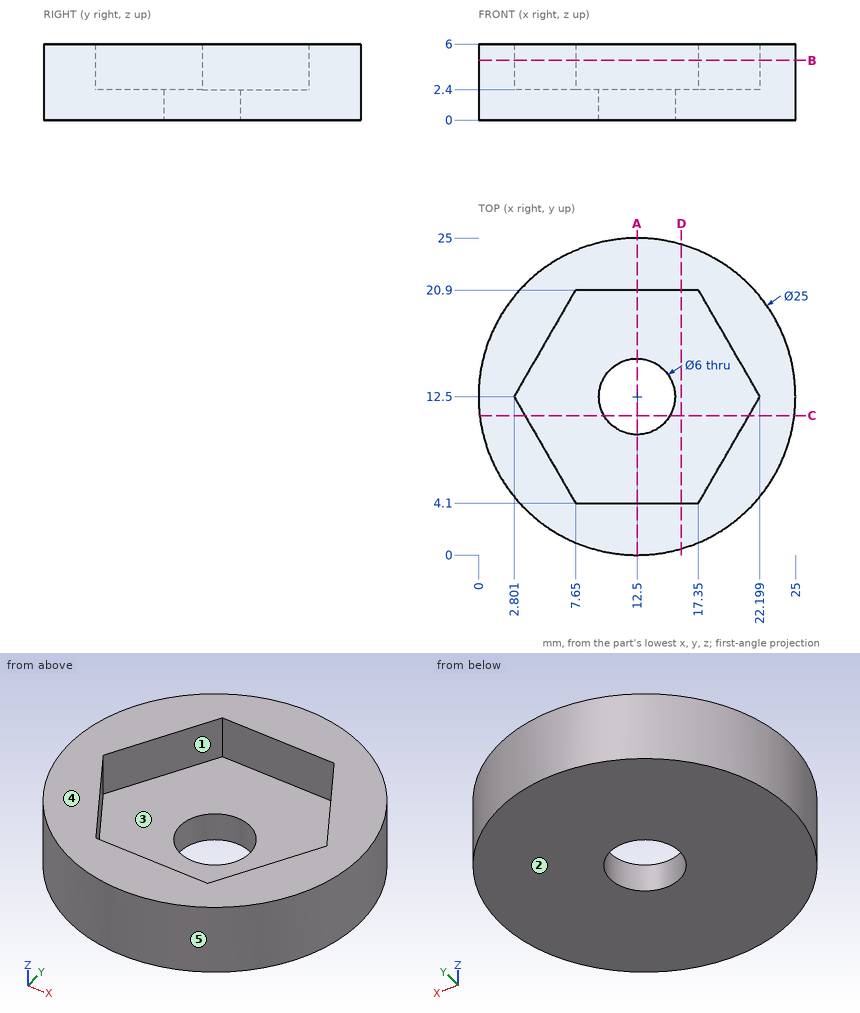
For this review, use the dimensioned drawing (mm, ordinates from the lowest corner) and the shaded views. A direction names the side the tool comes from. Give positions to 0.01 mm unless a question says otherwise; leave off trailing zeros. Loops run counter-clockwise (first coordinate to the right, second up) from the corner with the lowest first, then second, coordinate; pieces in that order, holes last.
Item 1: Insertion check: pin 1 (2 mm diameter, centred on y = 5.5, z = 5, fed in from +X) (1 decimal); pin 2 (3 mm diameter, centred on x = 19.5, z = 5, fed in from +Y) (1 decimal); pin 3 (1 mm diameter, centred on y = 6.5, z = 4.5, fed in from -X) (1 decimal). Each pin has a flat end and moves straight along its axis. Give the tip position at first contact, or say it passes through.
Item 2: Take a section at C-C, the plane y = 11. State the section outline as (x, z) points.
Item 3: Take a section at B-B, the plane z = 4.7. State the section outline as (x, y) points.
Item 4: For line 1 along Y through (x, z) = (12.5, 0.55); line 2 along Z through (x, y) = (7.5, 19.5); line 3 along X through (y, z) = (3.25, 4.6) (1 decimal), list the stretches that pass through material, from the lowest coordinate up.
Item 5: Take a section at A-A, the plane x = 12.5. State the section outline as (y, z) points.
Item 6: Tool access review of the marked faces 1 and 2: name each direction out of +Z, -Z, +X, -X, +Y, -Y from which nothing blocks a thin tool from reaching the whole face with its end or side.
Item 7: Draft analysis for pull direction X (two halves, no side actions). For the marked faces 3, 4 and 5, state which applies: +X half, -X half, draft (parallel to the pull), parting line (faces both ways), or undercut.
Item 8: Take a section at D-D, the plane x = 16. State the section outline as (y, z) points.
Calculated:
1. pin 1: stops at x = 23.5
1. pin 2: stops at y = 23.7
1. pin 3: stops at x = 1.3
2. outline: (0.09, 0) - (9.9, 0) - (9.9, 2.4) - (3.67, 2.4) - (3.67, 6) - (0.09, 6) - close; (15.1, 0) - (24.91, 0) - (24.91, 6) - (21.33, 6) - (21.33, 2.4) - (15.1, 2.4) - close
3. outline: circle Ø25 at (12.5, 12.5); hole (2.8, 12.5) - (7.65, 4.1) - (17.35, 4.1) - (22.2, 12.5) - (17.35, 20.9) - (7.65, 20.9) - close
4. line 1: y = 0 to 9.5, 15.5 to 25
4. line 2: z = 0 to 2.4
4. line 3: x = 4.1 to 20.9
5. outline: (0, 0) - (9.5, 0) - (9.5, 2.4) - (4.1, 2.4) - (4.1, 6) - (0, 6) - close; (15.5, 0) - (25, 0) - (25, 6) - (20.9, 6) - (20.9, 2.4) - (15.5, 2.4) - close
6. face 1: +Z
6. face 2: -Z, +X, -X, +Y, -Y
7. face 3: undercut
7. face 4: draft
7. face 5: parting line
8. outline: (0.5, 0) - (24.5, 0) - (24.5, 6) - (20.9, 6) - (20.9, 2.4) - (4.1, 2.4) - (4.1, 6) - (0.5, 6) - close
